Could you check a few things on this model? Use its own coordinates, in mm. A direction names the side the tool comes from. Give positions to 0.01 mm unless a question says otherwise; leave off trailing zeros. Order: outer loops, then holes, each group sorted by start corner. A loop starts at its lowest first (then second) coordinate and runs counter-clockwise, first axis right, second up. Notation, with made-up numbers: (17, 7.25) -> (57, 7.25) arc R23 ccw to (57, 38.25) -> close; hole circle Ø5 at (60.25, 8.25). An arc over 180 degrees is marked (long way). Answer as CSV lines item,"result". Start each with the question number.
(1) On a 3-axis mill with a long thin cutter (end or side, diameter ignored), from which of +Z, -Z, +X, -X, +Y, -Y can I reach the whole of each face in a straight line? I mean faces 1 (the face through (28.217, -35, 58)), 2 (the face through (0, -27.662, 28)), 3 (the face through (-2, 60.112, 36)). Say none if no direction works.
(2) I want a section at D-D (z = 49.5). Please give me the cut outline in (x, y), plus the area to 3 significant figures.
(3) I want a section at B-B (z = 39). Please give me the cut outline in (x, y).
(4) I want a section at A-A (x = 65). Please give me the cut outline in (y, z).
(5) I need wall thicknesses on L1, parallel to Y at x = 30, z = 60; L2, parallel to X at y = -3.5, z = 18.5; L3, parallel to Y at x = -69, z = 46. Which ranges of each line are inside material? Lowest first, please.
(6) We'd pull the mould along X, two halves only. Please class faces 4 (the face through (-71.272, -3.354, 49.26)), 5 (the face through (74.999, 8, 36)), 6 (the face through (-2, 53, 43.045)): released by +X, released by -X, zero draft, split by the parting line, or undercut.
(7) Will this pin go through, and if not, where does the flat tip stop? pin 1 Ø11.5 at (x, y) = (-9, -34.5) entering from +Z.
(8) I want a section at C-C (y = 43.5). Please give me the cut outline in (x, z), plus the area to 3 significant figures.
```python
from build123d import *

# Parameters (mm, degrees)
F0_W     = 151.0983854532
F0_H     = 101.8927358091
F0_W_2   = 134.0441703796
F0_H_2   = 73.9419609308
F1_DEPTH = 72.898
F2_W     = 59.4862736762
F2_H     = 29.8526170533
F3_DEPTH = 161.29
F4_R     = 11.294462473
F5_DEPTH = 227.838


with BuildPart() as f1:
    # F0 (on Top) → F1 (new body)
    with BuildSketch(Plane.XY):
        with Locations((-0.5501508713, 9.1656837612)):
            Rectangle(F0_W, F0_H)
        with Locations((0.444740057, 9.3090310693)):
            Rectangle(F0_W_2, F0_H_2, mode=Mode.SUBTRACT)
    extrude(amount=F1_DEPTH)

    # F2 (on face) → F3 (cut)
    with BuildSketch(Plane.XZ.offset(41.7806841433)):
        with Locations((-1.5259776264, 57.9716914734)):
            Rectangle(F2_W, F2_H)
    extrude(amount=-F3_DEPTH, mode=Mode.SUBTRACT)

    # F4 (on face) → F5 (cut)
    with BuildSketch(Plane.YZ.offset(74.9990418553)):
        with Locations((5.608974956, 56.1325512826)):
            Circle(F4_R)
    extrude(amount=-F5_DEPTH, mode=Mode.SUBTRACT)


solid = f1.part
```
Final values:
1,face 1,"+Z, +Y, -Y"
1,face 2,"+Z, -Z"
1,face 3,"+Z, -Z, +X, -X, +Y"
2,outline,"(-76.1, -41.78) -> (-31.27, -41.78) -> (-31.27, -27.66) -> (-66.58, -27.66) -> (-66.58, -3.53) -> (-76.1, -3.53) -> close; (-76.1, 14.75) -> (-66.58, 14.75) -> (-66.58, 46.28) -> (-31.27, 46.28) -> (-31.27, 60.11) -> (-76.1, 60.11) -> close; (28.22, -41.78) -> (75, -41.78) -> (75, -3.53) -> (67.47, -3.53) -> (67.47, -27.66) -> (28.22, -27.66) -> close; (28.22, 46.28) -> (67.47, 46.28) -> (67.47, 14.75) -> (75, 14.75) -> (75, 60.11) -> (28.22, 60.11) -> close"
2,area,"3,510 mm²"
3,outline,"(-76.1, -41.78) -> (75, -41.78) -> (75, 60.11) -> (-76.1, 60.11) -> close; hole (-66.58, -27.66) -> (67.47, -27.66) -> (67.47, 46.28) -> (-66.58, 46.28) -> close"
4,outline,"(-41.78, 0) -> (-27.66, 0) -> (-27.66, 72.9) -> (-41.78, 72.9) -> close; (46.28, 0) -> (60.11, 0) -> (60.11, 72.9) -> (46.28, 72.9) -> close"
5,L1,"-41.78 to -27.66, 46.28 to 60.11"
5,L2,"-76.1 to -66.58, 67.47 to 75"
5,L3,"-41.78 to 0.62, 10.6 to 60.11"
6,face 4,"zero draft"
6,face 5,"released by +X"
6,face 6,"undercut"
7,pin 1,"z = 43.05"
8,outline,"(-76.1, 0) -> (-66.58, 0) -> (-66.58, 72.9) -> (-76.1, 72.9) -> close; (67.47, 0) -> (75, 0) -> (75, 72.9) -> (67.47, 72.9) -> close"
8,area,"1,240 mm²"
